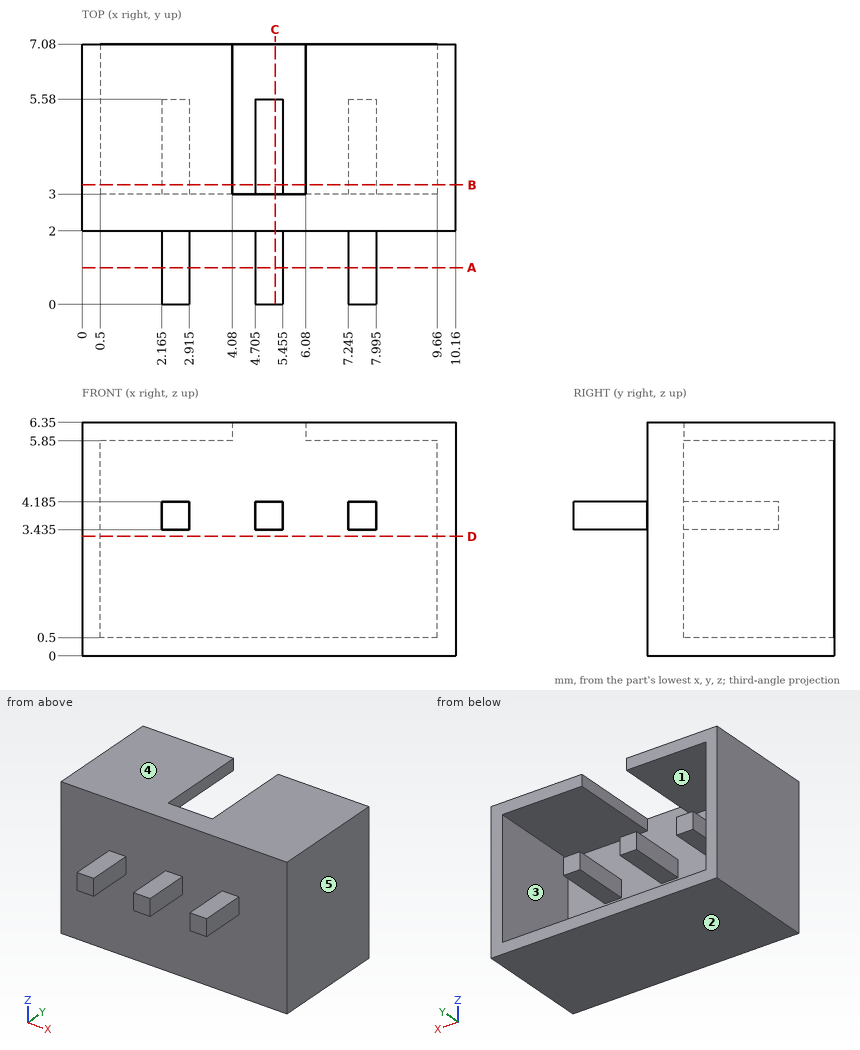
Can you work these out from the drawing? Everything is in mm from the part's minimum corner. A direction names the side the tool comes from. Round coordinates to 2 decimals unless told otherwise and drop trailing zeros. Write each loop counter-clockwise with the first axis right and the second up, starting at its lowest first coordinate (ties: lowest second). Pieces come first, ordered by that corner, then holes. Notation, with made-up numbers: M -13.5,40 L 33.5,40 A11 ccw 33.5,57 Z; hole C 86.5,24.5 d6. An arc over 180 degrees is marked long. Use a Markdown table: item, result.
Item 1: I want a section at C-C (x = 5.25). List the corners of the cut face in (y, z) for me (3 decimals).
Found:
| item | result |
|---|---|
| outline | M 0,3.435 L 2,3.435 L 2,0 L 7.08,0 L 7.08,0.5 L 3,0.5 L 3,3.435 L 5.58,3.435 L 5.58,4.185 L 3,4.185 L 3,6.35 L 2,6.35 L 2,4.185 L 0,4.185 Z |
Item 2: Which directions (+Z, -Z, +X, -X, +Y, -Y) give clear straight access to the entire face, cutting with the end or side of a thin tool? Please do the marked faces 1 and 2.
Found:
| item | result |
|---|---|
| face 1 | +Y |
| face 2 | -Z, +X, -X, +Y, -Y |
Item 3: If I drill on line 1 along X through (y, z) = (6.5, 4.25); line 2 along Z through (x, y) = (4, 5.5); line 3 along Z through (x, y) = (5, 4.5) (3 decimals), over which ranges is the centre line in solid material (lowest first)? Write a range as [from, to].
Found:
| item | result |
|---|---|
| line 1 | x = [0, 0.5], [9.66, 10.16] |
| line 2 | z = [0, 0.5], [5.85, 6.35] |
| line 3 | z = [0, 0.5], [3.435, 4.185] |
Item 4: For pin 1 Ø1.5 at (x, z) = (4, 3.5) entering from +Y; pin 2 Ø0.8 at (y, z) = (1, 3.5) entering from +X (3 decimals), each with a flat end and sliding along its axis, tell me the tip position at first contact or that it passes through.
Found:
| item | result |
|---|---|
| pin 1 | stops at y = 5.58 |
| pin 2 | stops at x = 7.995 |
Item 5: We'd pull the mould along X, two halves only. Please class the marked faces 3, 4 and 5: released by +X, released by -X, zero draft, split by the parting line, or undercut.
Found:
| item | result |
|---|---|
| face 3 | undercut |
| face 4 | zero draft |
| face 5 | released by +X |
Item 6: I want a section at D-D (z = 3.25). List the corners of the cut face in (x, y) for me, and give its area (3 significant figures).
Found:
| item | result |
|---|---|
| outline | M 0,2 L 10.16,2 L 10.16,7.08 L 9.66,7.08 L 9.66,3 L 0.5,3 L 0.5,7.08 L 0,7.08 Z |
| area | 14.2 mm2 |
Item 7: I want a section at B-B (y = 3.25). List the corners of the cut face in (x, z) for me (3 decimals), and give its area (3 significant figures).
Found:
| item | result |
|---|---|
| outline | M 0,0 L 10.16,0 L 10.16,6.35 L 6.08,6.35 L 6.08,5.85 L 9.66,5.85 L 9.66,0.5 L 0.5,0.5 L 0.5,5.85 L 4.08,5.85 L 4.08,6.35 L 0,6.35 Z; M 2.165,3.435 L 2.915,3.435 L 2.915,4.185 L 2.165,4.185 Z; M 4.705,3.435 L 5.455,3.435 L 5.455,4.185 L 4.705,4.185 Z; M 7.245,3.435 L 7.995,3.435 L 7.995,4.185 L 7.245,4.185 Z |
| area | 16.2 mm2 |
Item 8: I want a section at A-A (y = 1). List the corners of the cut face in (x, z) for me (3 decimals).
Found:
| item | result |
|---|---|
| outline | M 2.165,3.435 L 2.915,3.435 L 2.915,4.185 L 2.165,4.185 Z; M 4.705,3.435 L 5.455,3.435 L 5.455,4.185 L 4.705,4.185 Z; M 7.245,3.435 L 7.995,3.435 L 7.995,4.185 L 7.245,4.185 Z |
